Design review of the part built by this model. Coordinates are the model's own, in mm. A direction names the side the tool comes from. Give positions to 0.01 mm unless a question says otherwise; leave off trailing zeros. Order: outer loops, then holes, each group sorted by start corner. A loop starts at its lowest first (then second) coordinate and runs counter-clockwise, first axis right, second up. Notation, with made-up numbers: M -33.75,0 L 22.25,0 A32 cw 22.25,39 Z; hole C 38,29.5 d4. An arc over 180 degrees is marked long. Put each result on its own line as item: value. Start each with the question number.
from build123d import *

# Parameters (mm, degrees)
BOSS_EXTRUDE1_DEPTH = 3.175
SKETCH2_R           = 21.5
CUT_EXTRUDE1_DEPTH  = 215.322525648
SKETCH3_W           = 42
SKETCH3_H           = 55.35
SKETCH3_W_2         = 25
SKETCH3_H_2         = 96.35
CUT_EXTRUDE2_DEPTH  = 215.322525648
SKETCH4_R           = 1.5
CUT_EXTRUDE3_DEPTH  = 215.322525648
SKETCH5_R           = 2
CUT_EXTRUDE4_DEPTH  = 215.322525648
SKETCH7_R           = 1.55
CUT_EXTRUDE6_DEPTH  = 215.322525648
SKETCH8_W           = 25
SKETCH8_H           = 58.25
BOSS_EXTRUDE2_DEPTH = 6.35
FILLET1_R           = 2


with BuildPart() as part:
    # Sketch1 → Boss-Extrude1 (new, symmetric)
    with BuildSketch(Plane(origin=(0, 0, 0), x_dir=(1, 0, 0), z_dir=(0, 1, 0))):
        with BuildLine():
            ThreePointArc((35, 0), (0, 35), (-35, 0))
            Line((-35, 0), (-27.5, -211.35))
            Line((-27.5, -211.35), (27.5, -211.35))
            Line((27.5, -211.35), (35, 0))
        make_face()
    extrude(amount=BOSS_EXTRUDE1_DEPTH, both=True)

    # Sketch2 → Cut-Extrude1 (cut, through all)
    with BuildSketch(Plane(origin=(0, 3.175, 0), x_dir=(1, 0, 0), z_dir=(0, 1, 0))):
        with Locations(Location((0, 0, 0), (0, 0, 270))):
            Circle(SKETCH2_R)
    extrude(amount=-CUT_EXTRUDE1_DEPTH, mode=Mode.SUBTRACT)

    # Sketch3 → Cut-Extrude2 (cut, through all)
    with BuildSketch(Plane(origin=(0, 3.175, 0), x_dir=(1, 0, 0), z_dir=(0, 1, 0))):
        with Locations((0, -87.325)):
            Rectangle(SKETCH3_W, SKETCH3_H)
        with Locations((0, -163.175)):
            Rectangle(SKETCH3_W_2, SKETCH3_H_2)
    extrude(amount=-CUT_EXTRUDE2_DEPTH, mode=Mode.SUBTRACT)

    # Sketch4 → Cut-Extrude3 (cut, through all)
    with BuildSketch(Plane(origin=(0, 3.175, 0), x_dir=(1, 0, 0), z_dir=(0, 1, 0))):
        with Locations(Location((-19.35, 19.35, 0), (0, 0, 270))):
            Circle(SKETCH4_R)
        with Locations(Location((19.35, 19.35, 0), (0, 0, 270))):
            Circle(SKETCH4_R)
        with Locations(Location((19.35, -19.35, 0), (0, 0, 270))):
            Circle(SKETCH4_R)
        with Locations(Location((-19.35, -19.35, 0), (0, 0, 270))):
            Circle(SKETCH4_R)
    extrude(amount=-CUT_EXTRUDE3_DEPTH, mode=Mode.SUBTRACT)

    # Sketch5 → Cut-Extrude4 (cut, through all)
    with BuildSketch(Plane(origin=(0, 3.175, 0), x_dir=(1, 0, 0), z_dir=(0, 1, 0))):
        with Locations(Location((-20, -195, 0), (0, 0, 270))):
            Circle(SKETCH5_R)
        with Locations(Location((20, -195, 0), (0, 0, 270))):
            Circle(SKETCH5_R)
        with Locations(Location((20, -125, 0), (0, 0, 90))):
            Circle(SKETCH5_R)
        with Locations(Location((-20, -125, 0), (0, 0, 90))):
            Circle(SKETCH5_R)
    extrude(amount=-CUT_EXTRUDE4_DEPTH, mode=Mode.SUBTRACT)

    # Sketch7 → Cut-Extrude6 (cut, through all)
    with BuildSketch(Plane.XZ.offset(3.175)):
        with Locations(Location((-20, 206.35, 0), (0, 0, 270))):
            Circle(SKETCH7_R)
        with Locations(Location((20, 206.35, 0), (0, 0, 270))):
            Circle(SKETCH7_R)
    extrude(amount=-CUT_EXTRUDE6_DEPTH, mode=Mode.SUBTRACT)

    # Sketch8 → Boss-Extrude2 (add)
    with BuildSketch(Plane(origin=(0, 3.175, 0), x_dir=(1, 0, 0), z_dir=(0, 1, 0))):
        with Locations((0, -169.525)):
            Rectangle(SKETCH8_W, SKETCH8_H)
    extrude(amount=-BOSS_EXTRUDE2_DEPTH)

    # Fillet1
    fillet1_edges = [part.edges().sort_by_distance(p)[0] for p in [
        (-12.5, 0, 198.65),
        (12.5, 0, 198.65),
        (-21, 0, 59.65),
        (21, 0, 59.65),
    ]]
    fillet(fillet1_edges, radius=FILLET1_R)


solid = part.part
1. To check wall thickness, follow probe 1 along X at (y, z) = (1.5, 0); probe 2 along X at (y, z) = (0.25, 19.35); probe 3 along X at (y, z) = (0.5, 125). State the ranges of each line that lie inside material, in increasing order.
2. Insertion check: pin 1 (3 mm diameter, centred on y = 1.5, z = 101, fed in from +X); pin 2 (3 mm diameter, centred on y = 0, z = 126.5, fed in from -X); pin 3 (3 mm diameter, centred on y = 0.5, z = 91, fed in from -X). Each pin has a flat end and moves straight along its axis. Give the tip position at first contact, or say it passes through.
3. Machinability: for faces 4 (the flat face through (-12.5, 0, 206)), 5 (the flat face through (0, 0, 140.4)), 6 (the flat face through (23, -3.175, 86)), which of the approach directions +Z, -Z, +X, -X, +Y, -Y give a long, thin tool a straight path to every point of the face, cutting with its end or side? Answer none if there is none.
4. Consider section C-C on z = 109. Give the boundary of the cut face in (x, y) (3 decimals), then the cut area to 3 significant figures.
5. The part is to be moulded in two halves that separate along Z. For faces 1 (the flat face through (-21, 0, 89)), 2 (the flat face through (20, 0, 211.35)), 3 (the flat face through (23, 3.175, 86)), say which applies: +Z half, -Z half, draft (parallel to the pull), parting line (faces both ways), or undercut.
6. Consider section B-B on y = -2. Give the number of separate pieces and of enclosed holes in the cut face, then the cut area to 3 significant figures.
7. Consider section D-D on x = 31. Give the boundary of the cut face in (y, z) (3 decimals), then the cut area to 3 significant figures.
8. Consider section A-A on x = 0. Give the boundary of the cut face in (y, z) (3 decimals).
Returned:
1. probe 1: x = -35 to -21.5, 21.5 to 35
1. probe 2: x = -34.31 to -20.85, -17.85 to -9.37, 9.37 to 17.85, 20.85 to 34.31
1. probe 3: x = -30.56 to -22, -18 to -12.5, 12.5 to 18, 22 to 30.56
2. pin 1: stops at x = 31.47
2. pin 2: stops at x = -30.56
2. pin 3: stops at x = -31.82
3. face 4: +Z, +Y, -Y
3. face 5: +Y, -Y
3. face 6: +Z, -Z, +X, -X, -Y
4. outline: M -31.132,-3.175 L -21,-3.175 L -21,3.175 L -31.132,3.175 Z; M 21,-3.175 L 31.132,-3.175 L 31.132,3.175 L 21,3.175 Z
4. area: 129 mm2
5. face 1: undercut
5. face 2: +Z half
5. face 3: draft
6. separate pieces: 1
6. enclosed holes: 12
6. area: 10,300 mm2
7. outline: M -3.175,-16.248 L 3.175,-16.248 L 3.175,112.72 L -3.175,112.72 Z
7. area: 819 mm2
8. outline: M -3.175,-35 L 3.175,-35 L 3.175,-21.5 L -3.175,-21.5 Z; M -3.175,21.5 L 3.175,21.5 L 3.175,59.65 L -3.175,59.65 Z; M -3.175,140.4 L 3.175,140.4 L 3.175,198.65 L -3.175,198.65 Z
